Could you check a few things on this model? Use its own coordinates, in mm. A direction names the side the tool comes from. Coordinates: 2 decimals unless noted, no trailing zeros. Loops run counter-clockwise (first coordinate to the right, second up) from the corner with the lowest first, then second, coordinate; pieces in that order, holes last.
1) Thinking about a two-plate mould opening in X: for faces 5 (the face through (20.59, 17.45, -7.9)), 6 (the face through (-36.89, 18.5, 8.97)), 7 (the face through (21, 19, -5.4)), 8 (the face through (37.9, 10, 0)), which applies, released by +X, released by -X, zero draft, split by the parting line, or undercut?
2) Imagine slicing it at C-C on x = 0. Please give me the cut outline in (y, z).
3) Imagine slicing it at D-D on x = -28.5. Please give me the cut outline in (y, z).
4) Imagine slicing it at A-A on y = 14. Please give me the cut outline in (x, z), plus the area to 3 significant figures.
5) Imagine slicing it at B-B on z = 0. Please give me the cut outline in (x, y), plus the area to 3 significant figures.
6) If I drill on line 1 along X through (y, z) = (1, 0); line 2 along Z through (x, y) = (25, 3); line 3 along X through (y, z) = (18, 0), over which ranges is the centre line in solid material (lowest first)?
7) Will these pins go through, and if not, where does the flat tip stop? P1, Ø2, axis at x = -23.5, z = 2.5, coming from the +Y side; P2, Ø0.8, axis at x = 4, z = 9.5, coming from the +Y side; P3, Ø1, axis at x = -26.5, z = 7, coming from the +Y side.
8) For faces 1 (the face through (-1, 8, -10.4)), 2 (the face through (9.5, 16, 9)), 3 (the face through (-1, 7, 8.9)), 4 (the face through (-21, 19, 5.4)), which set-ups out of +Z, -Z, +X, -X, +Y, -Y let a thin tool reach every point of the face, with its end or its side?
```python
from build123d import *

# Parameters (mm, degrees)
CROQUIS1_W                        = 75.8
CROQUIS1_H                        = 20.8
SALIENTE_EXTRUIR1_DEPTH           = 20
REDONDEO1_R                       = 5
REDONDEO2_R                       = 0.5
VACIADO1_START                    = -36.4
VACIADO1_DEPTH                    = 72.8
CORTAR_EXTRUIR1_DEPTH             = 45.097278828
CORTAR_EXTRUIR1_DEPTH_BACK        = 45.097278828
CORTAR_EXTRUIR2_REACH             = 45.438
CROQUIS3_R                        = 1.75
CORTAR_EXTRUIR2_DIRECTION_2_DEPTH = 44.437541367


# Read off the part's stored shape, not the designer's step: Vaciado1
with BuildPart() as part:
    # Croquis1 → Saliente-Extruir1 (new body)
    with BuildSketch(Plane(origin=(0, 0, 0), x_dir=(1, 0, 0), z_dir=(0, 1, 0))):
        Rectangle(CROQUIS1_W, CROQUIS1_H)
    extrude(amount=SALIENTE_EXTRUIR1_DEPTH)

    # Redondeo1
    redondeo1_edges = [part.edges().sort_by_distance(p)[0] for p in [
        (0, 20, 10.4),
        (0, 20, -10.4),
    ]]
    fillet(redondeo1_edges, radius=REDONDEO1_R)

    # Redondeo2
    redondeo2_edges = [part.edges().sort_by_distance(p)[0] for p in [
        (37.9, 20, 0),
        (-37.9, 20, 0),
        (-37.9, 7.5, 10.4),
        (-37.9, 7.5, -10.4),
        (-37.9, 18.535533906, 8.935533906),
        (-37.9, 18.535533906, -8.935533906),
        (37.9, 7.5, -10.4),
        (37.9, 7.5, 10.4),
        (37.9, 18.535533906, 8.935533906),
        (37.9, 18.535533906, -8.935533906),
        (0, 0, 10.4),
        (-37.9, 0, 0),
        (0, 0, -10.4),
        (37.9, 0, 0),
    ]]
    fillet(redondeo2_edges, radius=REDONDEO2_R)

    # Vaciado1 outline → Vaciado1 (cut)
    with BuildSketch(Plane.YZ.offset(VACIADO1_START)):
        with BuildLine():
            Line((20, -5.4), (20, 5.4))
            Line((20, 5.4), (18.5, 5.4))
            ThreePointArc((18.5, 5.4), (17.474873734, 7.874873734), (15, 8.9))
            Line((15, 8.9), (1.5, 8.9))
            Line((1.5, 8.9), (1.5, -8.9))
            Line((1.5, -8.9), (15, -8.9))
            ThreePointArc((15, -8.9), (17.474873734, -7.874873734), (18.5, -5.4))
            Line((18.5, -5.4), (20, -5.4))
        make_face()
    extrude(amount=VACIADO1_DEPTH, mode=Mode.SUBTRACT)

    # Croquis2 → Cortar-Extruir1 (cut, two sides: drawn at the far end of the back side and taken through both)
    with BuildSketch(Plane.XY.offset(-CORTAR_EXTRUIR1_DEPTH_BACK)):
        Polygon((-9.5, 11), (9.5, 11), (9.5, 20), (32, 20), (32, 11), (36.4, 11), (36.4, 23), (-36.4, 23), (-36.4, 11), (-32, 11), (-32, 20), (-9.5, 20), align=None)
    extrude(amount=CORTAR_EXTRUIR1_DEPTH + CORTAR_EXTRUIR1_DEPTH_BACK, mode=Mode.SUBTRACT)

    # Croquis3 → Cortar-Extruir2 (cut, up to next)
    with BuildSketch(Plane(origin=(0, 1.5, 0), x_dir=(1, 0, 0), z_dir=(0, 1, 0)), mode=Mode.PRIVATE) as cortar_extruir2_sk1:
        with Locations(Location((0, 0, 0), (0, 0, 270))):
            Circle(CROQUIS3_R)
    cortar_extruir2_tool1 = extrude(cortar_extruir2_sk1.sketch, amount=-CORTAR_EXTRUIR2_REACH, mode=Mode.PRIVATE) & part.part
    add(cortar_extruir2_tool1.solids().sort_by_distance((0, 1.5, 0))[0], mode=Mode.SUBTRACT)

    # Croquis3 → Cortar-Extruir2 direction 2 (cut)
    with BuildSketch(Plane(origin=(0, 1.5, 0), x_dir=(1, 0, 0), z_dir=(0, 1, 0))):
        with Locations(Location((0, 0, 0), (0, 0, 270))):
            Circle(CROQUIS3_R)
    extrude(amount=CORTAR_EXTRUIR2_DIRECTION_2_DEPTH, mode=Mode.SUBTRACT)


solid = part.part
```
Filled in:
1. face 5: undercut
1. face 6: zero draft
1. face 7: undercut
1. face 8: released by +X
2. outline: (0, -9.9) arc R0.5 ccw to (0.5, -10.4) - (11, -10.4) - (11, -8.9) - (1.5, -8.9) - (1.5, -1.75) - (0, -1.75) - close; (0, 1.75) - (1.5, 1.75) - (1.5, 8.9) - (11, 8.9) - (11, 10.4) - (0.5, 10.4) arc R0.5 ccw to (0, 9.9) - close
3. outline: (0, -9.9) arc R0.5 ccw to (0.5, -10.4) - (15, -10.4) arc R5 ccw to (20, -5.4) - (18.5, -5.4) arc R3.5 cw to (15, -8.9) - (1.5, -8.9) - (1.5, 8.9) - (15, 8.9) arc R3.5 cw to (18.5, 5.4) - (20, 5.4) arc R5 ccw to (15, 10.4) - (0.5, 10.4) arc R0.5 ccw to (0, 9.9) - close
4. outline: (-37.9, -9.9) arc R0.5 ccw to (-37.4, -10.4) - (-36.4, -10.4) - (-36.4, 10.4) - (-37.4, 10.4) arc R0.5 ccw to (-37.9, 9.9) - close; (-32, -10.4) - (-9.5, -10.4) - (-9.5, -8.9) - (-32, -8.9) - close; (-32, 8.9) - (-9.5, 8.9) - (-9.5, 10.4) - (-32, 10.4) - close; (9.5, -10.4) - (32, -10.4) - (32, -8.9) - (9.5, -8.9) - close; (9.5, 8.9) - (32, 8.9) - (32, 10.4) - (9.5, 10.4) - close; (36.4, -10.4) - (37.4, -10.4) arc R0.5 ccw to (37.9, -9.9) - (37.9, 9.9) arc R0.5 ccw to (37.4, 10.4) - (36.4, 10.4) - close
4. area: 197 mm2
5. outline: (-37.9, 0.5) arc R0.5 ccw to (-37.4, 0) - (-1.75, 0) - (-1.75, 1.5) - (-36.4, 1.5) - (-36.4, 20) - (-37.4, 20) arc R0.5 ccw to (-37.9, 19.5) - close; (1.75, 0) - (37.4, 0) arc R0.5 ccw to (37.9, 0.5) - (37.9, 19.5) arc R0.5 ccw to (37.4, 20) - (36.4, 20) - (36.4, 1.5) - (1.75, 1.5) - close
5. area: 164 mm2
6. line 1: x = -37.9 to -1.75, 1.75 to 37.9
6. line 2: z = -10.4 to -8.9, 8.9 to 10.4
6. line 3: x = -37.9 to -36.4, 36.4 to 37.9
7. P1: stops at y = 1.5
7. P2: stops at y = 11
7. P3: stops at y = 19.88
8. face 1: -Z, +X, -X, +Y, -Y
8. face 2: +Z, -Z, +Y
8. face 3: none
8. face 4: +Y
